The model under review builds one solid part; all positions refer to its coordinate system, in mm. A direction names the side the tool comes from. Round coordinates to 2 decimals unless told otherwise and drop trailing zeros. Order: outer loops, then holes, each group sorted by start corner. A loop starts at its lowest first (then second) coordinate and runs counter-clockwise, first axis right, second up. Notation, with made-up numbers: M -13.5,89 L -7.5,89 A31 cw -7.5,127 Z; hole C -33,20 d6. An arc over 180 degrees is marked long. Use a Markdown table: item, result. Add a question column.
1. Consider section D-D on z = -19. State the section outline as (x, y) points.
2. Consider section A-A on y = 8.75. State the section outline as (x, z) points.
3. Consider section B-B on z = -48.5. State the section outline as (x, y) points, then the cut area to 3 significant figures.
4. To check wall thickness, follow probe 1 along Z at (x, y) = (72, 8.5); probe 2 along X at (y, z) = (9.5, -75); probe 3 along Z at (x, y) = (90.5, 17.75). State the ranges of each line that lie inside material, in increasing order.
5. Consider section C-C on x = 83.5. State the section outline as (y, z) points, then the cut area to 3 significant figures.
6. The part is to be moulded in two halves that separate along X. For faces 1 (the flat face through (54, 10, -110)), 2 (the flat face through (110, 10, -54)), 3 (the flat face through (20.28, 12.36, -55.7)), say which applies: +X half, -X half, draft (parallel to the pull), parting line (faces both ways), or undercut.
7. Insertion check: P1, Ø8, axis at x = 94.5, z = -52.5, coming from the +Y side; P2, Ø8, axis at x = 16.5, z = -96, coming from the +Y side. Each pin has a flat end and moves straight along its axis. Give the tip position at first contact, or say it passes through.
8. For faces 4 (the flat face through (0, 10, -54)), 5 (the flat face through (56, 12, -89)), list the 3-axis set-ups (+Z, -Z, +X, -X, +Y, -Y) from which the entire face can be reached by the end or side of a thin tool; tool diameter is ignored.
from build123d import *

# Parameters (mm, degrees)
CROQUIS1_W                          = 110
CROQUIS1_H                          = 110
CROQUIS1_W_2                        = 100
CROQUIS1_H_2                        = 100
SALIENTE_EXTRUIR1_DEPTH             = 20
SALIENTE_EXTRUIR2_DEPTH             = 100
SALIENTE_EXTRUIR3_REACH             = 126.599
SALIENTE_EXTRUIR3_DIRECTION_2_REACH = 126.599


with BuildPart() as part:
    # Croquis1 → Saliente-Extruir1 (new body)
    with BuildSketch(Plane(origin=(0, 0, 0), x_dir=(1, 0, 0), z_dir=(0, 1, 0))):
        with Locations((55, 55)):
            Rectangle(CROQUIS1_W, CROQUIS1_H)
        with Locations((55, 55)):
            Rectangle(CROQUIS1_W_2, CROQUIS1_H_2, mode=Mode.SUBTRACT)
    extrude(amount=SALIENTE_EXTRUIR1_DEPTH)

    # Croquis2 → Saliente-Extruir2 (add)
    with BuildSketch(Plane.XY.offset(-105)):
        Polygon((5, 20), (45, 0), (5, 0), align=None)
        Polygon((105, 0), (105, 20), (65, 0), align=None)
    extrude(amount=SALIENTE_EXTRUIR2_DEPTH)

    # Saliente-Extruir3: up to this face of the body (flat: up to its plane)
    saliente_extruir3_end = Plane(part.part.faces().sort_by_distance((110, 10, -55))[0])
    # Croquis3 → Saliente-Extruir3 (add, up to the picked face)
    with BuildSketch(Plane(origin=(55, 0, 0), x_dir=(0, 0, -1), z_dir=(1, 0, 0)), mode=Mode.PRIVATE) as saliente_extruir3_sk1:
        Polygon((5, 20), (45, 0), (5, 0), align=None)
    saliente_extruir3_tool1 = split(extrude(saliente_extruir3_sk1.sketch, amount=SALIENTE_EXTRUIR3_REACH, mode=Mode.PRIVATE), bisect_by=saliente_extruir3_end, keep=Keep.BOTH, mode=Mode.PRIVATE)
    # Croquis3 → Saliente-Extruir3 (add, up to the picked face)
    with BuildSketch(Plane(origin=(55, 0, 0), x_dir=(0, 0, -1), z_dir=(1, 0, 0)), mode=Mode.PRIVATE) as saliente_extruir3_sk2:
        Polygon((105, 0), (65, 0), (105, 20), align=None)
    saliente_extruir3_tool2 = split(extrude(saliente_extruir3_sk2.sketch, amount=SALIENTE_EXTRUIR3_REACH, mode=Mode.PRIVATE), bisect_by=saliente_extruir3_end, keep=Keep.BOTH, mode=Mode.PRIVATE)
    add(saliente_extruir3_tool1.solids().sort_by(Axis((55, 6.666667, -18.333333), (1, 0, 0)))[0])
    add(saliente_extruir3_tool2.solids().sort_by(Axis((55, 6.666667, -91.666667), (1, 0, 0)))[0])

    # Saliente-Extruir3 direction 2: up to this face of the body (flat: up to its plane)
    saliente_extruir3_direction_2_end = Plane(part.part.faces().sort_by_distance((0, 10, -55))[0])
    # Croquis3 → Saliente-Extruir3 direction 2 (add, up to the picked face)
    with BuildSketch(Plane(origin=(55, 0, 0), x_dir=(0, 0, -1), z_dir=(1, 0, 0)), mode=Mode.PRIVATE) as saliente_extruir3_direction_2_sk1:
        Polygon((5, 20), (45, 0), (5, 0), align=None)
    saliente_extruir3_direction_2_tool1 = split(extrude(saliente_extruir3_direction_2_sk1.sketch, amount=-SALIENTE_EXTRUIR3_DIRECTION_2_REACH, mode=Mode.PRIVATE), bisect_by=saliente_extruir3_direction_2_end, keep=Keep.BOTH, mode=Mode.PRIVATE)
    # Croquis3 → Saliente-Extruir3 direction 2 (add, up to the picked face)
    with BuildSketch(Plane(origin=(55, 0, 0), x_dir=(0, 0, -1), z_dir=(1, 0, 0)), mode=Mode.PRIVATE) as saliente_extruir3_direction_2_sk2:
        Polygon((105, 0), (65, 0), (105, 20), align=None)
    saliente_extruir3_direction_2_tool2 = split(extrude(saliente_extruir3_direction_2_sk2.sketch, amount=-SALIENTE_EXTRUIR3_DIRECTION_2_REACH, mode=Mode.PRIVATE), bisect_by=saliente_extruir3_direction_2_end, keep=Keep.BOTH, mode=Mode.PRIVATE)
    add(saliente_extruir3_direction_2_tool1.solids().sort_by(Axis((55, 6.666667, -18.333333), (-1, 0, 0)))[0])
    add(saliente_extruir3_direction_2_tool2.solids().sort_by(Axis((55, 6.666667, -91.666667), (-1, 0, 0)))[0])


solid = part.part
Answer block:
| question | item | result |
|---|---|---|
| 1 | outline | M 0,0 L 110,0 L 110,20 L 105,20 L 91,13 L 19,13 L 5,20 L 0,20 Z |
| 2 | outline | M 0,-110 L 110,-110 L 110,0 L 0,0 Z; hole M 27.5,-82.5 L 82.5,-82.5 L 82.5,-27.5 L 27.5,-27.5 Z |
| 3 | outline | M 0,0 L 45,0 L 5,20 L 0,20 Z; M 65,0 L 110,0 L 110,20 L 105,20 Z |
| 3 | area | 1,000 mm^2 |
| 4 | probe 1 | -110 to -82, -28 to 0 |
| 4 | probe 2 | 0 to 26, 84 to 110 |
| 4 | probe 3 | -110 to -100.5, -9.5 to 0 |
| 5 | outline | M 0,-110 L 20,-110 L 20,-105 L 9.25,-83.5 L 9.25,-26.5 L 20,-5 L 20,0 L 0,0 Z |
| 5 | area | 1,360 mm^2 |
| 6 | face 1 | draft |
| 6 | face 2 | +X half |
| 6 | face 3 | undercut |
| 7 | P1 | y = 16.75 |
| 7 | P2 | y = 17.5 |
| 8 | face 4 | +Z, -Z, -X, +Y, -Y |
| 8 | face 5 | +Y |
